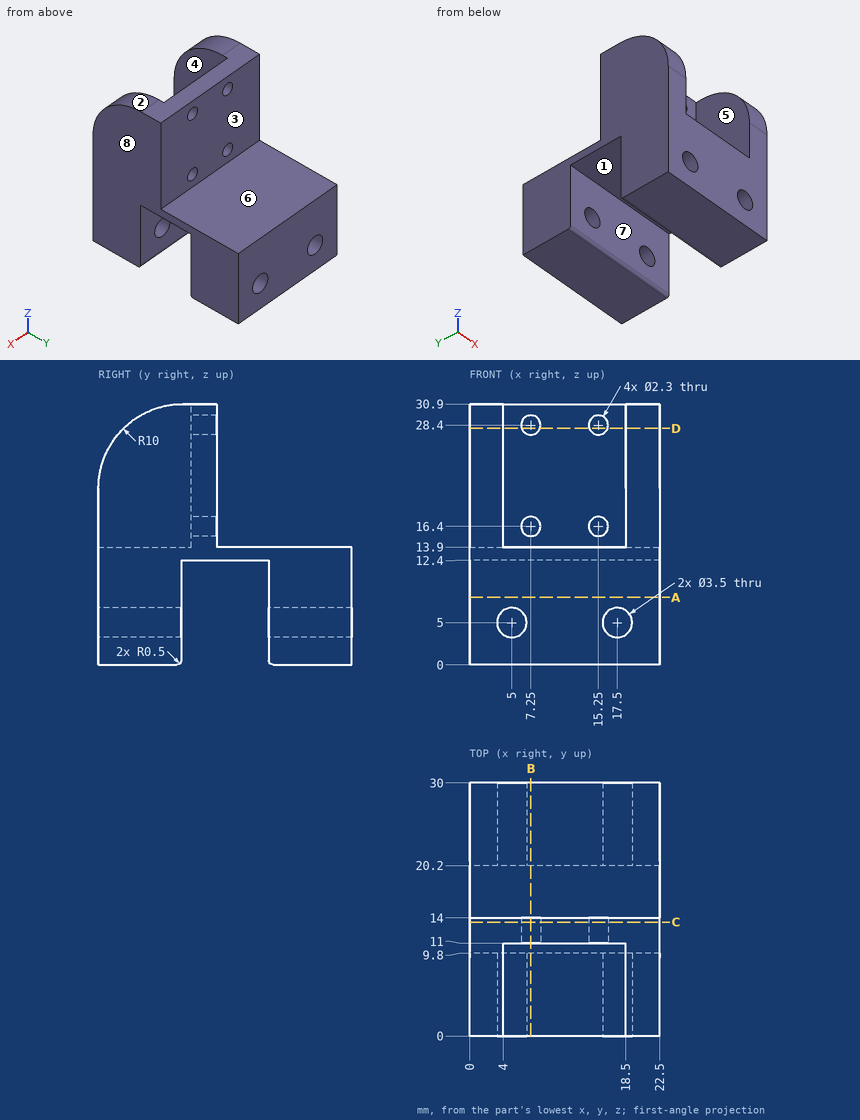
Source: three-view drawing plus pictorial views. Frame: mm from the lowest corner of the part. A direction names the side the tool comes from. Round coordinates to 2 decimals unless told otherwise and drop trailing zeros. Order: outer loops, then holes, each group sorted by start corner. A loop starts at its lowest first (then second) coordinate and runs counter-clockwise, first axis right, second up. Notation, with made-up numbers: (44, 60) - (67, 60) arc R20 ccw to (67, 84) - close; hole circle Ø2 at (88.25, -29). An arc over 180 degrees is marked (long way). Answer in a Markdown table with one row per item.
Item 1: Line query: line 1 (X direction, y = 12.5, z = 28.4); line 2 (X direction, y = 3.75, z = 5); line 3 (Z direction, x = 15.25, y = 11.85). Output: solid intervals per line, ascending.
Model answer:
| item | result |
|---|---|
| line 1 | x = 0 to 6.1, 8.4 to 14.1, 16.4 to 22.5 |
| line 2 | x = 0 to 3.25, 6.75 to 15.75, 19.25 to 22.5 |
| line 3 | z = 12.4 to 15.25, 17.55 to 27.25, 29.55 to 30.9 |
Item 2: Section query A-A (z = 8). Return the cut outline in (x, y).
Model answer:
| item | result |
|---|---|
| outline | (0, 0) - (22.5, 0) - (22.5, 9.8) - (0, 9.8) - close; (0, 20.2) - (22.5, 20.2) - (22.5, 30) - (0, 30) - close |
Item 3: Mould query, pull axis Y, two halves, no side actions, for the marked faces 1, 2, 3 and 4. Classes: released by +Y, released by -Y, zero draft, split by the parting line, or undercut.
Model answer:
| item | result |
|---|---|
| face 1 | undercut |
| face 2 | released by -Y |
| face 3 | released by +Y |
| face 4 | zero draft |
Item 4: Section query B-B (x = 7.25). Return the cut outline in (y, z).
Model answer:
| item | result |
|---|---|
| outline | (0, 0) - (9.3, 0) arc R0.5 ccw to (9.8, 0.5) - (9.8, 12.4) - (20.2, 12.4) - (20.2, 0.5) arc R0.5 ccw to (20.7, 0) - (30, 0) - (30, 13.9) - (14, 13.9) - (14, 15.25) - (11, 15.25) - (11, 13.9) - (0, 13.9) - close; (11, 17.55) - (14, 17.55) - (14, 27.25) - (11, 27.25) - close; (11, 29.55) - (14, 29.55) - (14, 30.9) - (11, 30.9) - close |
Item 5: Pin query (flat end, axial travel): pin 1 (8 mm diameter, centred on x = 12, y = 16, fed in from +Z); pin 2 (8 mm diameter, centred on x = 13, y = 21.5, fed in from +Z); pin 3 (7 mm diameter, centred on x = 12, z = 19.5, fed in from -Y); pin 4 (5 mm diameter, centred on x = 9.5, y = 13.5, fed in from -Z). Return the tip coordinate at first contact, or that it passes through.
Model answer:
| item | result |
|---|---|
| pin 1 | stops at z = 30.9 |
| pin 2 | stops at z = 13.9 |
| pin 3 | stops at y = 11 |
| pin 4 | stops at z = 12.4 |
Item 6: Reachability of the marked faces 5, 6, 7 and 8 from +Z, -Z, +X, -X, +Y, -Y: full face, straight path, thin tool, end or side. Return the list, or none.
Model answer:
| item | result |
|---|---|
| face 5 | +Z, -Y |
| face 6 | +Z, +X, -X, +Y |
| face 7 | -Z, +X, -X |
| face 8 | +Z, -Z, +X, +Y, -Y |
Item 7: Section query D-D (z = 28). Return the cut outline in (x, y).
Model answer:
| item | result |
|---|---|
| outline | (0, 2.96) - (4, 2.96) - (4, 11) - (6.17, 11) - (6.17, 14) - (0, 14) - close; (8.33, 11) - (14.17, 11) - (14.17, 14) - (8.33, 14) - close; (16.33, 11) - (18.5, 11) - (18.5, 2.96) - (22.5, 2.96) - (22.5, 14) - (16.33, 14) - close |
Item 8: Section query C-C (y = 13.5). Return the cut outline in (x, z), then the cut area to 3 significant figures.
Model answer:
| item | result |
|---|---|
| outline | (0, 12.4) - (22.5, 12.4) - (22.5, 30.9) - (0, 30.9) - close; hole circle Ø2.3 at (7.25, 16.4); hole circle Ø2.3 at (7.25, 28.4); hole circle Ø2.3 at (15.25, 16.4); hole circle Ø2.3 at (15.25, 28.4) |
| area | 400 mm² |
